```python
from build123d import *

# Parameters (mm, degrees)
EXTRUDE_1_DEPTH     = 150
SKETCH_2_R          = 25
EXTRUDE_2_DEPTH     = 300
SKETCH_3_R          = 25
CUT_EXTRUDE_1_DEPTH = 300


with BuildPart() as part:
    # 스케치1 → 보스-돌출1 (new body)
    with BuildSketch(Plane(origin=(0, 0, 0), x_dir=(1, 0, 0), z_dir=(0, 1, 0))):
        Polygon((-100, -100), (-150, -100), (-150, 100), (150, 100), (150, -100), (100, -100), (100, 80), (-100, 80), align=None)
    extrude(amount=EXTRUDE_1_DEPTH)

    # 스케치2 → 보스-돌출2 (add)
    with BuildSketch(Plane(origin=(0, 0, -100), x_dir=(-1, 0, 0), z_dir=(0, 0, -1))):
        with Locations((0, 75)):
            Circle(SKETCH_2_R)
    extrude(amount=EXTRUDE_2_DEPTH)

    # 스케치3 → 컷-돌출1 (cut)
    with BuildSketch(Plane.ZY.offset(150)):
        with Locations((50, 75)):
            Circle(SKETCH_3_R)
    extrude(amount=-CUT_EXTRUDE_1_DEPTH, mode=Mode.SUBTRACT)


solid = part.part
```
Here's how the part is built. I have some questions about the finished solid (model axes, mm). A direction names the side the tool comes from. Coordinates: 2 decimals unless noted, no trailing zeros. Write each loop counter-clockwise with the first axis right and the second up, starting at its lowest first coordinate (ties: lowest second). Pieces come first, ordered by that corner, then holes. Notation, with made-up numbers: (-30.5, 50.5) - (3.5, 50.5) arc R10 ccw to (3.5, 59.5) - close; hole circle Ø4 at (35, -25.75). An arc over 180 degrees is marked (long way). One line per item, written item: value.
1) Suppose I cut it at D-D on x = 0. Write out the boundary of the cut face in (y, z), and give its area (3 significant figures).
Model answer:
outline: (0, -100) - (50, -100) - (50, -400) - (100, -400) - (100, -100) - (150, -100) - (150, -80) - (0, -80) - close
area: 18,000 mm²
2) We'd pull the mould along X, two halves only. Please class faces 4 (the flat face through (125, 74, 100)), 5 (the flat face through (-100, 74, 9)), 6 (the flat face through (-150, 74, 1)), 7 (the flat face through (1, 74, -80)): pulls with the +X half, pulls with the -X half, needs draft (parallel to the pull), parting line crosses it, or undercut.
Model answer:
face 4: needs draft
face 5: undercut
face 6: pulls with the -X half
face 7: undercut
3) Suppose I cut it at A-A on z = -21.5. Write out the boundary of the cut face in (x, y), and give its area (3 significant figures).
Model answer:
outline: (-150, 0) - (-100, 0) - (-100, 150) - (-150, 150) - close; (100, 0) - (150, 0) - (150, 150) - (100, 150) - close
area: 15,000 mm²
4) I need wall thicknesses on line 1 along X through (y, z) = (34, 4); line 2 along Y through (x, z) = (-110.5, 50); line 3 along Z through (x, y) = (-130.5, 48). Which ranges of each line are inside material? Lowest first, please.
Model answer:
line 1: x = -150 to -100, 100 to 150
line 2: y = 0 to 50, 100 to 150
line 3: z = -100 to 100
5) I'm going to push flat-ended pins straight in: P1, Ø12, axis at x = 70, y = 127, coming from the -Z side; P2, Ø5, axis at x = -3, z = -107, coming from the -Y side (3 decimals); P3, Ø1.5, axis at x = 3, z = -303, coming from the -Y side. Where does each tip first touch, or does it pass through?
Model answer:
P1: stops at z = -100
P2: stops at y = 50.005
P3: stops at y = 50.1
6) On a 3-axis mill with a long thin cutter (end or side, diameter ignored), from which of +Z, -Z, +X, -X, +Y, -Y can I reach the whole of each face in a straight line? I mean faces 1 (the cylindrical face through (124.65, 50.594, 44.58)), 2 (the cylindrical face through (5.42, 50.594, -247.9)), 3 (the flat face through (100, 74, 11)). Say none if no direction works.
Model answer:
face 1: +X, -X
face 2: -Z
face 3: +Z, +Y, -Y
7) Suppose I cut it at C-C on z = 50. Write out the boundary of the cut face in (x, y), and give its area (3 significant figures).
Model answer:
outline: (-150, 0) - (-100, 0) - (-100, 50) - (-150, 50) - close; (-150, 100) - (-100, 100) - (-100, 150) - (-150, 150) - close; (100, 0) - (150, 0) - (150, 50) - (100, 50) - close; (100, 100) - (150, 100) - (150, 150) - (100, 150) - close
area: 10,000 mm²
8) Suppose I cut it at B-B on y = 75. Write out the boundary of the cut face in (x, z), and give its area (3 significant figures).
Model answer:
outline: (-150, -100) - (-25, -100) - (-25, -400) - (25, -400) - (25, -100) - (150, -100) - (150, 25) - (100, 25) - (100, -80) - (-100, -80) - (-100, 25) - (-150, 25) - close; (-150, 75) - (-100, 75) - (-100, 100) - (-150, 100) - close; (100, 75) - (150, 75) - (150, 100) - (100, 100) - close
area: 34,000 mm²
